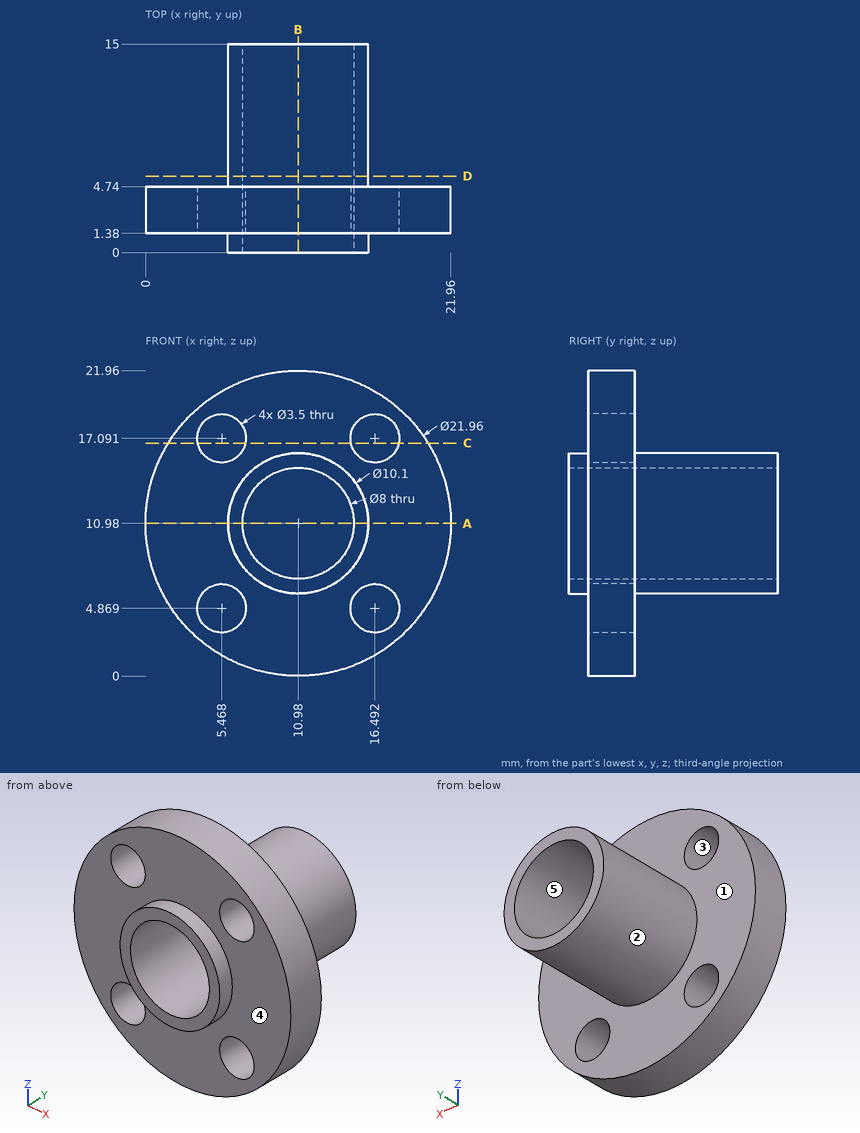
For this review, use the dimensioned drawing (mm, ordinates from the lowest corner) and the shaded views. A direction names the side the tool comes from. Round coordinates to 2 decimals unless told otherwise and drop trailing zeros. Order: outer loops, then holes, each group sorted by start corner. A loop starts at its lowest first (then second) coordinate and runs counter-clockwise, first axis right, second up. Notation, with made-up numbers: M 47,20 L 79,20 A22 cw 79,31 Z; hole C -14.5,-28 d10. An arc over 180 degrees is marked long. Use a Markdown table: item, result.
1) Insertion check: pin 1 (3 mm diameter, centred on y = 2.5, z = 15.5, fed in from +X); pin 2 (2 mm diameter, centred on x = 5.47, z = 17.09, fed in from -Y); pin 3 (1 mm diameter, centred on x = 3, z = 16.5, fed in from -Y). Each pin has a flat end and moves straight along its axis. Give the tip position at first contact, or say it passes through.
Report:
| item | result |
|---|---|
| pin 1 | x = 21.54 |
| pin 2 | through |
| pin 3 | y = 1.38 |
2) Draft analysis for pull direction X (two halves, no side actions). For the marked faces 1, 2 and 3, state which applies: released by +X, released by -X, zero draft, split by the parting line, or undercut.
Report:
| item | result |
|---|---|
| face 1 | zero draft |
| face 2 | split by the parting line |
| face 3 | undercut |
3) Wall thickness on line 1 along Y through (x, z) = (19.25, 4.25); line 2 along Z through (x, y) = (12.5, 11.25) (1 decimal); line 3 along X through (y, z) = (2.5, 6.25) (1 decimal): over which ranges is each line inside the solid? List them lowest first. Write a range as [from, to].
Report:
| item | result |
|---|---|
| line 1 | [1.38, 4.74] |
| line 2 | [6.2, 7.3], [14.7, 15.8] |
| line 3 | [1.1, 4.4], [6.5, 15.4], [17.6, 20.9] |
4) Consider section C-C (z = 16.75). Write out the cut boundary in (x, y) (1 decimal).
Report:
| item | result |
|---|---|
| outline | M 1.6,1.4 L 3.8,1.4 L 3.8,4.7 L 1.6,4.7 Z; M 7.2,1.4 L 14.8,1.4 L 14.8,4.7 L 7.2,4.7 Z; M 18.2,1.4 L 20.3,1.4 L 20.3,4.7 L 18.2,4.7 Z |
5) Consider section B-B (x = 10.98). Write out the cut boundary in (y, z).
Report:
| item | result |
|---|---|
| outline | M 0,5.93 L 1.38,5.93 L 1.38,0 L 4.74,0 L 4.74,5.93 L 15,5.93 L 15,6.98 L 0,6.98 Z; M 0,14.98 L 15,14.98 L 15,16.03 L 4.74,16.03 L 4.74,21.96 L 1.38,21.96 L 1.38,16.03 L 0,16.03 Z |
6) Consider section A-A (z = 10.98). Write out the cut boundary in (x, y).
Report:
| item | result |
|---|---|
| outline | M 0,1.38 L 5.93,1.38 L 5.93,0 L 6.98,0 L 6.98,15 L 5.93,15 L 5.93,4.74 L 0,4.74 Z; M 14.98,0 L 16.03,0 L 16.03,1.38 L 21.96,1.38 L 21.96,4.74 L 16.03,4.74 L 16.03,15 L 14.98,15 Z |
7) Tool access review of the marked faces 4 and 5: name each direction out of +Z, -Z, +X, -X, +Y, -Y from which nothing blocks a thin tool from reaching the whole face with its end or side.
Report:
| item | result |
|---|---|
| face 4 | -Y |
| face 5 | +Y, -Y |
8) Consider section D-D (y = 5.5). Write out the cut boundary in (x, z).
Report:
| item | result |
|---|---|
| outline | C 10.98,10.98 d10.1; hole C 10.98,10.98 d8 |
